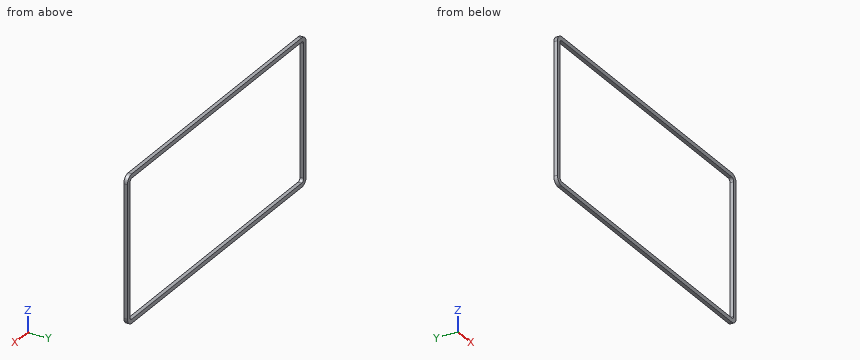
Autodesk Inventor part; units mm, degrees
ref_plane "YZ Plane" through (0, 0, 0) normal (1, 0, 0) x (0, 1, 0)
ref_plane "XZ Plane" through (0, 0, 0) normal (0, 1, 0) x (-1, 0, 0)
ref_plane "XY Plane" through (0, 0, 0) normal (0, 0, 1) x (1, 0, 0)
sketch "Sketch1" plane through (0, 0, 0) normal (0, 1, 0) x (-1, 0, 0)
  line L0 (3.175, 0) -> (123.825, 0)
  line L1 (127, -3.175) -> (127, -60.325)
  line L2 (123.825, -63.5) -> (3.175, -63.5)
  line L3 (0, -60.325) -> (0, -3.175)
  arc A0 (127, -3.175) -> (123.825, 0) centre (123.825, -3.175) ccw
  arc A1 (123.825, -63.5) -> (127, -60.325) centre (123.825, -60.325) ccw
  arc A2 (0, -60.325) -> (3.175, -63.5) centre (3.175, -60.325) ccw
  arc A3 (3.175, 0) -> (0, -3.175) centre (3.175, -3.175) ccw
  line L4 (1.905, -3.175) -> (1.905, -60.325)
  arc A4 (1.905, -60.325) -> (3.175, -61.595) centre (3.175, -60.325) ccw
  line L5 (3.175, -61.595) -> (123.825, -61.595)
  arc A5 (123.825, -61.595) -> (125.095, -60.325) centre (123.825, -60.325) ccw
  line L6 (125.095, -60.325) -> (125.095, -3.175)
  arc A6 (125.095, -3.175) -> (123.825, -1.905) centre (123.825, -3.175) ccw
  line L7 (123.825, -1.905) -> (3.175, -1.905)
  arc A7 (3.175, -1.905) -> (1.905, -3.175) centre (3.175, -3.175) ccw
  line L8 (3.175, -1.778) -> (123.825, -1.778)
  arc A8 (125.222, -3.175) -> (123.825, -1.778) centre (123.825, -3.175) ccw
  line L9 (125.222, -3.175) -> (125.222, -60.325)
  arc A9 (123.825, -61.722) -> (125.222, -60.325) centre (123.825, -60.325) ccw
  line L10 (123.825, -61.722) -> (3.175, -61.722)
  arc A10 (1.778, -60.325) -> (3.175, -61.722) centre (3.175, -60.325) ccw
  line L11 (1.778, -60.325) -> (1.778, -3.175)
  arc A11 (3.175, -1.778) -> (1.778, -3.175) centre (3.175, -3.175) ccw
  point P0 (0, 0)
  point P1 (127, -63.5)
  point P2 (127, 0)
  point P3 (0, -63.5)
  point P4 (3.175, -3.175)
  point P5 (123.825, -3.175)
  point P6 (123.825, -60.325)
  point P7 (3.175, -60.325)
  dimension "d0" = 63.5
  dimension "d1" = 127
  dimension "d2" = 3.175
  dimension "d3" = 3.175
  dimension "d7" = 1.905
  dimension "d12" = 0.127
extrude "Extrusion1" add sketch "Sketch1" along normal blind 1.5875 contours L0 A0 L1 A1 L2 A2 L3 A3
equation "\"d3\" = d2"
properties part number "PinecilCaseBorder" material "ABS Plastic"
Here's how the part is built. I have some questions about the finished solid (model axes, mm). Coordinates: 2 decimals unless noted, no trailing zeros. Loops run counter-clockwise (first coordinate to the right, second up) from the corner with the lowest first, then second, coordinate; pieces in that order, holes last. Notation, with made-up numbers: M 10,67 L 55,67 A29 cw 55,97 Z; hole C 13,-19.75 d7. An arc over 180 degrees is marked long. One line per item, written item: value.
1. Imagine slicing it at C-C (y = 0.95). List the corners of the cut face in (x, z) for me (3 decimals).
Geometry says:
outline: M -127,-60.325 A3.175 ccw -123.825,-63.5 L -3.175,-63.5 A3.175 ccw 0,-60.325 L 0,-3.175 A3.175 ccw -3.175,0 L -123.825,0 A3.175 ccw -127,-3.175 Z; hole M -125.222,-60.325 A1.397 ccw -123.825,-61.722 L -3.175,-61.722 A1.397 ccw -1.778,-60.325 L -1.778,-3.175 A1.397 ccw -3.175,-1.778 L -123.825,-1.778 A1.397 ccw -125.222,-3.175 Z
2. Imagine slicing it at A-A (z = -47.5). List the corners of the cut face in (x, y) for me, and give its area (3 significant figures).
Geometry says:
outline: M -127,0 L -125.22,0 L -125.22,1.59 L -127,1.59 Z; M -1.78,0 L 0,0 L 0,1.59 L -1.78,1.59 Z
area: 5.65 mm2
3. Will these pins go through, and if not, where does the flat tip stop? pin 1 Ø12 at (x, z) = (-59, -54) entering from +Y; pin 2 Ø0.5 at (y, z) = (0.5, -21.5) entering from +X.
Geometry says:
pin 1: passes through
pin 2: stops at x = 0
4. Imagine slicing it at B-B (x = -106). List the corners of the cut face in (y, z) for me, and give its area (3 significant figures).
Geometry says:
outline: M 0,-63.5 L 1.59,-63.5 L 1.59,-61.72 L 0,-61.72 Z; M 0,-1.78 L 1.59,-1.78 L 1.59,0 L 0,0 Z
area: 5.65 mm2
5. Please list where these lines run through material, in increasing order: probe 1 along X at (y, z) = (0.8, -34.5); probe 2 along Z at (x, y) = (-90, 1.4).
Geometry says:
probe 1: x = -127 to -125.22, -1.78 to 0
probe 2: z = -63.5 to -61.72, -1.78 to 0
